Source: CAD feature listing. Evaluate the final solid. Frame: model axes, mm. A direction names the side the tool comes from. Coordinates: 2 decimals unless noted, no trailing zeros. Loops run counter-clockwise (first coordinate to the right, second up) from the corner with the lowest first, then second, coordinate; pieces in that order, holes last.
Item 1: Section query D-D, the plane y = 22.5. Return the cut outline in (x, z).
Item 2: Line query: probe 1 along Y at (x, z) = (0, 12.5) (1 decimal); probe 2 along Y at (x, z) = (-13.5, 1.5) (3 decimals); probe 3 along Y at (x, z) = (1, 15.5) (3 decimals). Output: solid intervals per line, ascending.
Item 3: Section query B-B, the plane y = 6. Return the cut outline in (x, z), then the cut area to 3 significant figures.
Item 4: Reachability of faces 1 (the flat face through (4.762, 60, 0)), 2 (the cylindrical face through (-6.3, 56.4, 0.8)), 3 (the flat face through (0, 29.145, 0)) from +Z, -Z, +X, -X, +Y, -Y: full face, straight path, thin tool, end or side. Return the list, or none.
Item 5: Pull-direction query (Y, two-part tool) for faces 4 (the cylindrical face through (4.722, 10.145, -14.667)), 5 (the cylindrical face through (1.431, 4.982, 14.543)), 6 (the flat face through (5, 47.625, -5)), 7 (the cylindrical face through (10.602, 24.085, 12.58)); classes: +Y half, -Y half, draft (parallel to the pull), parting line (faces both ways), or undercut.
Item 6: Pin query (flat end, axial travel): pin 1 Ø11.5 at (x, z) = (-7, 1.5) entering from +Y (3 decimals); pin 2 Ø6 at (x, z) = (7, -5.5) entering from -Y; pin 3 Ø5 at (y, z) = (13.5, -13.5) entering from +X (3 decimals); pin 4 Ø7 at (y, z) = (15.5, -14) entering from -X (3 decimals). Return the tip coordinate at first contact, or that it passes through.
Item 7: Section query A-A, the plane x = 0. State how many separate pieces and enclosed holes the cut face has, then the cut area to 3 significant figures.
```python
from build123d import *

# Parameters (mm, degrees)
SKETCH1_R               = 19.05
BASE_EXTRUDE_DEPTH      = 47.625
CUT_EXTRUDE1_DEPTH      = 55.716959208
CUT_EXTRUDE1_DEPTH_BACK = 55.716959208
CUT_EXTRUDE5_DEPTH      = 47.625
CUT_EXTRUDE5_DEPTH_BACK = 55.716959365
SKETCH8_W               = 20.32
SKETCH8_H               = 36.600526062
CUT_EXTRUDE6_DEPTH      = 55.716959365
CUT_EXTRUDE6_DEPTH_BACK = 55.716959365
SKETCH11_R              = 4.7625
SKETCH12_R              = 6.35
BOSS_EXTRUDE1_DEPTH     = 19.05
CHAMFER3_SIZE           = 1.27
CHAMFER3_SIZE2          = 2.199704526
CUT_EXTRUDE7_START      = -12.7
CUT_EXTRUDE7_DEPTH      = 12.7


with BuildPart() as part:
    # Sketch1 → Base-Extrude (new body)
    with BuildSketch(Plane(origin=(0, 0, 0), x_dir=(-1, 0, 0), z_dir=(0, 1, 0))):
        with Locations(Location((0, 0, 0), (0, 0, 90))):
            Circle(SKETCH1_R)
    extrude(amount=BASE_EXTRUDE_DEPTH)

    # Sketch2 → Cut-Extrude1 (cut, two sides: drawn at the far end of the back side and taken through both)
    with BuildSketch(Plane.XY.offset(-CUT_EXTRUDE1_DEPTH_BACK)):
        with BuildLine():
            Line((9.525, 9.525), (9.525, 19.685))
            ThreePointArc((9.525, 19.685), (12.314807909, 26.420192091), (19.05, 29.21))
            Line((19.05, 29.21), (19.05, -1.366191125))
            Line((19.05, -1.366191125), (-19.05, -1.366191125))
            Line((-19.05, -1.366191125), (-19.05, 29.21))
            ThreePointArc((-19.05, 29.21), (-12.314807909, 26.420192091), (-9.525, 19.685))
            Line((-9.525, 19.685), (-9.525, 9.525))
            ThreePointArc((-9.525, 9.525), (0, 0), (9.525, 9.525))
        make_face()
    extrude(amount=CUT_EXTRUDE1_DEPTH + CUT_EXTRUDE1_DEPTH_BACK, mode=Mode.SUBTRACT)

    # Sketch8 → Cut-Extrude5 (cut, two sides: drawn at the far end of the back side and taken through both)
    with BuildSketch(Plane(origin=(0, 0, 0), x_dir=(0, 0, -1), z_dir=(1, 0, 0)).offset(-CUT_EXTRUDE5_DEPTH_BACK)):
        with Locations((0, 10.844975795)):
            Rectangle(SKETCH8_W, SKETCH8_H)
    extrude(amount=CUT_EXTRUDE5_DEPTH + CUT_EXTRUDE5_DEPTH_BACK, mode=Mode.SUBTRACT)

    # Sketch11 → Cut-Extrude6 (cut, two sides: drawn at the far end of the back side and taken through both)
    with BuildSketch(Plane.XY.offset(-CUT_EXTRUDE6_DEPTH_BACK)):
        with Locations(Location((0, 9.525, 0), (0, 0, 270))):
            Circle(SKETCH11_R)
    extrude(amount=CUT_EXTRUDE6_DEPTH + CUT_EXTRUDE6_DEPTH_BACK, mode=Mode.SUBTRACT)

    # Sketch12 → Boss-Extrude1 (add)
    with BuildSketch(Plane(origin=(0, 47.625, 0), x_dir=(-1, 0, 0), z_dir=(0, 1, 0))):
        with Locations(Location((0, 0, 0), (0, 0, 270))):
            Circle(SKETCH12_R)
    extrude(amount=BOSS_EXTRUDE1_DEPTH)

    # Chamfer3
    chamfer3_edges = [part.edges().sort_by_distance(p)[0] for p in [
        (0, 66.675, 6.35),
    ]]
    chamfer3_side = [part.faces().sort_by_distance(p)[0] for p in [
        (0, 57.15, 6.35),
    ]]
    chamfer(chamfer3_edges, length=CHAMFER3_SIZE, length2=CHAMFER3_SIZE2, reference=chamfer3_side[0])

    # Sketch13 → Cut-Extrude7 (cut)
    with BuildSketch(Plane(origin=(0, 66.675, 0), x_dir=(-1, 0, 0), z_dir=(0, 1, 0)).offset(CUT_EXTRUDE7_START)):
        with BuildLine():
            Line((-4.7625, 4.200130206), (-4.7625, -4.200130206))
            ThreePointArc((-4.7625, -4.200130206), (-6.35, 0), (-4.7625, 4.200130206))
        make_face()
    extrude(amount=CUT_EXTRUDE7_DEPTH, mode=Mode.SUBTRACT)


solid = part.part
```
Verdict:
1. outline: (-9.95, -16.24) arc R19.05 ccw to (9.95, -16.24) - (9.95, -10.16) - (-9.95, -10.16) - close; (-9.95, 10.16) - (9.95, 10.16) - (9.95, 16.24) arc R19.05 ccw to (-9.95, 16.24) - close
2. probe 1: y = 0 to 4.8, 14.3 to 47.6
2. probe 2: y = 29.145 to 47.625
2. probe 3: y = 0.053 to 4.869, 14.181 to 47.625
3. outline: (-8.85, -16.87) arc R19.05 ccw to (-3.2, -18.78) - (-3.2, -10.16) - (-8.85, -10.16) - close; (-8.85, 10.16) - (-3.2, 10.16) - (-3.2, 18.78) arc R19.05 ccw to (-8.85, 16.87) - close; (3.2, -18.78) arc R19.05 ccw to (8.85, -16.87) - (8.85, -10.16) - (3.2, -10.16) - close; (3.2, 10.16) - (8.85, 10.16) - (8.85, 16.87) arc R19.05 ccw to (3.2, 18.78) - close
3. area: 177 mm2
4. face 1: +Z, -Z, +X, +Y
4. face 2: +Y
4. face 3: +X, -X, -Y
5. face 4: undercut
5. face 5: undercut
5. face 6: +Y half
5. face 7: -Y half
6. pin 1: stops at y = 66.675
6. pin 2: stops at y = 29.15
6. pin 3: stops at x = 9.525
6. pin 4: stops at x = -9.525
7. separate pieces: 3
7. enclosed holes: 0
7. area: 1,290 mm2
